The listing builds one solid part. Answer for the finished solid, in the listing's coordinates (mm). A direction names the side the tool comes from. Give positions to 0.01 mm unless a question says otherwise; leave off trailing zeros. Order: outer loops, then holes, each group sorted by start corner. A loop starts at its lowest first (then second) coordinate and runs counter-clockwise, first axis right, second up. Notation, with made-up numbers: (39, -5.5) - (52, -5.5) arc R34 cw to (52, 31.5) - close; hole circle Ø5 at (-30, -15). An arc over 180 degrees is marked (long way). Use CSV: the item, a comma, the result in double quotes.
```python
from build123d import *

# Parameters (mm, degrees)
BOSS_EXTRUDE1_DEPTH = 10
SKETCH5_W           = 16
SKETCH5_H           = 16
CUT_EXTRUDE1_DEPTH  = 120
CUT_EXTRUDE2_REACH  = 136.536
SKETCH3_W           = 16
SKETCH3_H           = 16
CUT_EXTRUDE3_DEPTH  = 2
FILLET1_R           = 2
FILLET2_R           = 2
FILLET3_R           = 2
FILLET4_R           = 2


with BuildPart() as part:
    # Sketch2 → Boss-Extrude1 (new, symmetric)
    with BuildSketch(Plane.XY):
        with BuildLine():
            Line((10, 60), (-10, 60))
            Line((-10, 60), (-10, 14))
            ThreePointArc((-10, 14), (-11.171572875, 11.171572875), (-14, 10))
            Line((-14, 10), (-60, 10))
            Line((-60, 10), (-60, -10))
            Line((-60, -10), (-14, -10))
            ThreePointArc((-14, -10), (-11.171572875, -11.171572875), (-10, -14))
            Line((-10, -14), (-10, -60))
            Line((-10, -60), (10, -60))
            Line((10, -60), (10, -14))
            ThreePointArc((10, -14), (11.171572875, -11.171572875), (14, -10))
            Line((14, -10), (60, -10))
            Line((60, -10), (60, 10))
            Line((60, 10), (14, 10))
            ThreePointArc((14, 10), (11.171572875, 11.171572875), (10, 14))
            Line((10, 14), (10, 60))
        make_face()
    extrude(amount=BOSS_EXTRUDE1_DEPTH, both=True)

    # Sketch5 → Cut-Extrude1 (cut)
    with BuildSketch(Plane(origin=(0, 60, 0), x_dir=(1, 0, 0), z_dir=(0, 1, 0))):
        Rectangle(SKETCH5_W, SKETCH5_H)
    extrude(amount=-CUT_EXTRUDE1_DEPTH, mode=Mode.SUBTRACT)

    # Cut-Extrude2: up to this face of the body (flat: up to its plane)
    cut_extrude2_end = Plane(part.part.faces().sort_by_distance((-60, 0, 0))[0])
    # Sketch3 → Cut-Extrude2 (cut, up to the picked face)
    with BuildSketch(Plane(origin=(60, 0, 0), x_dir=(0, 0, -1), z_dir=(1, 0, 0)), mode=Mode.PRIVATE) as cut_extrude2_sk1:
        Rectangle(SKETCH3_W, SKETCH3_H)
    cut_extrude2_tool1 = split(extrude(cut_extrude2_sk1.sketch, amount=-CUT_EXTRUDE2_REACH, mode=Mode.PRIVATE), bisect_by=cut_extrude2_end, keep=Keep.BOTH, mode=Mode.PRIVATE)
    add(cut_extrude2_tool1.solids().sort_by(Axis((60, 0, 0), (-1, 0, 0)))[0], mode=Mode.SUBTRACT)

    # Sketch6 → Cut-Extrude3 (cut)
    with BuildSketch(Plane.XY.offset(10)):
        with BuildLine():
            Line((-2, 4), (-2, 50))
            Line((-2, 50), (2, 50))
            Line((2, 50), (2, 4))
            ThreePointArc((2, 4), (2.585786438, 2.585786438), (4, 2))
            Line((4, 2), (50, 2))
            Line((50, 2), (50, -2))
            Line((50, -2), (4, -2))
            ThreePointArc((4, -2), (2.585786438, -2.585786438), (2, -4))
            Line((2, -4), (2, -50))
            Line((2, -50), (-2, -50))
            Line((-2, -50), (-2, -4))
            ThreePointArc((-2, -4), (-2.585786438, -2.585786438), (-4, -2))
            Line((-4, -2), (-50, -2))
            Line((-50, -2), (-50, 2))
            Line((-50, 2), (-4, 2))
            ThreePointArc((-4, 2), (-2.585786438, 2.585786438), (-2, 4))
        make_face()
    extrude(amount=-CUT_EXTRUDE3_DEPTH, mode=Mode.SUBTRACT)

    # Fillet1
    fillet1_edges = [part.edges().sort_by_distance(p)[0] for p in [
        (-2, 50, 9),
        (2, 50, 9),
    ]]
    fillet(fillet1_edges, radius=FILLET1_R - 0.0001)  # a hair under: the kernel refuses the full size

    # Fillet2
    fillet2_edges = [part.edges().sort_by_distance(p)[0] for p in [
        (2, -50, 9),
        (-2, -50, 9),
    ]]
    fillet(fillet2_edges, radius=FILLET2_R - 0.0001)  # a hair under: the kernel refuses the full size

    # Fillet3
    fillet3_edges = [part.edges().sort_by_distance(p)[0] for p in [
        (50, 2, 9),
        (50, -2, 9),
    ]]
    fillet(fillet3_edges, radius=FILLET3_R - 0.0001)  # a hair under: the kernel refuses the full size

    # Fillet4
    fillet4_edges = [part.edges().sort_by_distance(p)[0] for p in [
        (-50, -2, 9),
        (-50, 2, 9),
    ]]
    fillet(fillet4_edges, radius=FILLET4_R - 0.0001)  # a hair under: the kernel refuses the full size


solid = part.part
```
Item 1: The part is cut by section B-B (y = -52). Give the vertices of the cut face in (x, z), and give its area (3 significant figures).
Taken from the geometry:
outline,"(-10, -10) - (10, -10) - (10, 10) - (-10, 10) - close; hole (-8, -8) - (8, -8) - (8, 8) - (-8, 8) - close"
area,"144 mm^2"
Item 2: Find the intervals of material crossed by line 1 along X through (y, z) = (-32, 8.25); line 2 along Z through (x, y) = (6, 47.5), in increasing order.
Taken from the geometry:
line 1,"-10 to -2, 2 to 10"
line 2,"-10 to -8, 8 to 10"
Item 3: The part is cut by section C-C (z = 5.5). Give the vertices of the cut face in (x, y).
Taken from the geometry:
outline,"(-60, -10) - (-14, -10) arc R4 cw to (-10, -14) - (-10, -60) - (-8, -60) - (-8, -8) - (-60, -8) - close; (-60, 8) - (-8, 8) - (-8, 60) - (-10, 60) - (-10, 14) arc R4 cw to (-14, 10) - (-60, 10) - close; (8, -60) - (10, -60) - (10, -14) arc R4 cw to (14, -10) - (60, -10) - (60, -8) - (8, -8) - close; (8, 8) - (60, 8) - (60, 10) - (14, 10) arc R4 cw to (10, 14) - (10, 60) - (8, 60) - close"
Item 4: The mould has two halves that part along X. Classify faces 1 (the face through (-11.203, -11.141, 0.14)), 2 (the face through (-5, 5, 8)), 3 (the face through (37, -10, 0)): +X half, -X half, draft (parallel to the pull), parting line (faces both ways), or undercut.
Taken from the geometry:
face 1,"-X half"
face 2,"undercut"
face 3,"draft"
Item 5: Each of these flat-tipped pins is pushed along its axis until it touches: pin 1 (10 mm diameter, centred on y = 4.5, z = 7, fed in from -X); pin 2 (12 mm diameter, centred on x = -18, z = -1, fed in from -Y); pin 3 (5 mm diameter, centred on x = -35, z = 5.5, fed in from -Y); pin 4 (2 mm diameter, centred on y = 30.5, z = 9, fed in from +X). Where does it stop, or does it pass through?
Taken from the geometry:
pin 1,"x = -60"
pin 2,"y = -10.54"
pin 3,"y = -10"
pin 4,"x = 10"
Item 6: Which of the six approach directions +Z, -Z, +X, -X, +Y, -Y give full straight-line access (tool end or side, diameter ignored) to faces 4 (the face through (10, -37, 0)), 5 (the face through (-10, 37, 0)), 6 (the face through (-37, -10, 0)), 7 (the face through (8, -34, 0)), 8 (the face through (34, 8, 0))?
Taken from the geometry:
face 4,"+Z, -Z, +X, -Y"
face 5,"+Z, -Z, -X, +Y"
face 6,"+Z, -Z, -X, -Y"
face 7,"+Y, -Y"
face 8,"+X, -X"
Item 7: The part is cut by section A-A (x = -6.5). Give the vertices of the cut face in (y, z), and give its area (3 significant figures).
Taken from the geometry:
outline,"(-60, -10) - (60, -10) - (60, -8) - (-60, -8) - close; (-60, 8) - (-2, 8) - (-2, 10) - (-60, 10) - close; (2, 8) - (60, 8) - (60, 10) - (2, 10) - close"
area,"472 mm^2"
